Read the model definition and answer for the solid it produces. Units are mm, in the model's axes. A direction names the side the tool comes from. Round coordinates to 2 decimals unless told otherwise and drop trailing zeros. Order: outer loops, then holes, each group sorted by start corner. A loop starts at its lowest first (then second) coordinate and runs counter-clockwise, first axis right, second up. Notation, with made-up numbers: (42.5, 1) -> (61.5, 1) arc R31 ccw to (61.5, 28) -> close; hole circle Ø7 at (10, -7). An arc over 180 degrees is marked (long way). Use a Markdown table: item, result. Add a question column.
1. Section B-B, the plane z = -30 is taken. Give the vertices of the cut face in (x, y), then the cut area to 3 significant figures.
2. Section C-C, the plane y = 9 is taken. Give the vertices of the cut face in (x, z), then the cut area to 3 significant figures.
3. Section A-A, the plane y = 33 is taken. Give the vertices of the cut face in (x, z), then the cut area to 3 significant figures.
4. Consider L1, parallel to X at y = 61.5, z = -33.5; L2, parallel to Z at x = 115, y = 70.5; L3, parallel to Z at x = 97, y = 15.5. Determine where each line is inside the solid, lowest interval first. Write a range as [from, to].
5. The mould has two halves that part along X. Classify faces 5 (the face through (73.73, 13.72, -3.94)), 6 (the face through (116, -9, -33)), 7 (the face through (92.58, 13.72, -3.94)), 8 (the face through (45.675, 13.782, -3.944)): +X half, -X half, draft (parallel to the pull), parting line (faces both ways), or undercut.
6. Given pin 1 (1.4 mm diameter, centred on x = 47, z = -4.5, fed in from +Y); pin 2 (1 mm diameter, centred on y = 43.5, z = -56.5, fed in from -X); pin 3 (4 mm diameter, centred on x = 115.5, z = -13.5, fed in from +Y); pin 4 (12 mm diameter, centred on x = 90.5, z = -15, fed in from -Y), each flat-ended and moving along its own axis, determine where each tip first touches the part or whether it passes through.
7. For faces 1 (the face through (116, 10.5, -16)), 2 (the face through (83.374, 13.782, -3.944)), 3 (the face through (117.71, 13.72, -3.94)), 4 (the face through (116, 76, -103.5)), determine the directions among +Z, -Z, +X, -X, +Y, -Y from which every point of the face is accessible in a straight line to the end or side of a thin tool.
```python
from build123d import *

# Parameters (mm, degrees)
BLANKSKE_W          = 120
BLANKSKE_H          = 16
BLANK_DEPTH         = 8
TOOTHCUTSIM_DEPTH   = 122.326007105
TEETHCUTS_COUNT     = 20
TEETHCUTS_PITCH     = 6.2831853
SKETCH1_W           = 8
SKETCH1_H           = 1
CUT_EXTRUDE1_DEPTH  = 122.326007105
BOSS_EXTRUDE2_DEPTH = 8
CUT_EXTRUDE2_DEPTH  = 183.738200713


with BuildPart() as part:
    # BlankSke → Blank (new body)
    with BuildSketch(Plane.XY):
        with Locations((60, 8)):
            Rectangle(BLANKSKE_W, BLANKSKE_H)
    extrude(amount=-BLANK_DEPTH)

    # TooCutSkeSim → ToothCutSim (cut, through all)
    with BuildSketch(Plane.XY):
        Polygon((0.861870739, 11.5), (-0.861870739, 11.5), (-2.508981637, 16.0254), (2.508981637, 16.0254), align=None)
    toothcutsim = extrude(amount=-TOOTHCUTSIM_DEPTH, mode=Mode.SUBTRACT)

    # TeethCuts: ToothCutSim ×20
    with Locations(*[(i * TEETHCUTS_PITCH, 0, 0) for i in range(1, TEETHCUTS_COUNT)]):
        add(toothcutsim, mode=Mode.SUBTRACT)

    # Sketch1 → Cut-Extrude1 (cut, through all)
    with BuildSketch(Plane(origin=(120, 0, 0), x_dir=(0, 0, -1), z_dir=(1, 0, 0))):
        with Locations((4, 0.5)):
            Rectangle(SKETCH1_W, SKETCH1_H)
    extrude(amount=-CUT_EXTRUDE1_DEPTH, mode=Mode.SUBTRACT)

    # Sketch2 → Boss-Extrude2 (add)
    with BuildSketch(Plane(origin=(120, 0, 0), x_dir=(0, 0, -1), z_dir=(1, 0, 0))):
        Polygon((8, 1), (23.5, 1), (23.5, -9), (43.5, -9), (103.5, 61), (103.5, 91), (23.5, 91), (23.5, 10.5), (8, 10.5), align=None)
    extrude(amount=-BOSS_EXTRUDE2_DEPTH)

    # Sketch3 → Cut-Extrude2 (cut, through all)
    with BuildSketch(Plane.XY):
        with BuildLine():
            Line((0, 1), (0, 11.5))
            ThreePointArc((0, 11.5), (0.43093537, 11.93093537), (0.861870739, 11.5))
            Line((0.861870739, 11.5), (2.499736794, 16))
            Line((2.499736794, 16), (3.783448506, 16))
            Line((3.783448506, 16), (5.421314561, 11.5))
            Line((5.421314561, 11.5), (7.145056039, 11.5))
            Line((7.145056039, 11.5), (8.782922094, 16))
            Line((8.782922094, 16), (10.066633806, 16))
            Line((10.066633806, 16), (11.704499861, 11.5))
            Line((11.704499861, 11.5), (13.428241339, 11.5))
            Line((13.428241339, 11.5), (15.066107394, 16))
            Line((15.066107394, 16), (15.70796325, 16))
            Line((15.70796325, 16), (16.349819106, 16))
            Line((16.349819106, 16), (17.987685161, 11.5))
            Line((17.987685161, 11.5), (19.711426639, 11.5))
            Line((19.711426639, 11.5), (21.349292694, 16))
            Line((21.349292694, 16), (22.633004406, 16))
            Line((22.633004406, 16), (24.270870461, 11.5))
            Line((24.270870461, 11.5), (25.994611939, 11.5))
            Line((25.994611939, 11.5), (27.632477994, 16))
            Line((27.632477994, 16), (28.916189706, 16))
            Line((28.916189706, 16), (30.554055761, 11.5))
            Line((30.554055761, 11.5), (32.277797239, 11.5))
            Line((32.277797239, 11.5), (33.915663294, 16))
            Line((33.915663294, 16), (35.199375006, 16))
            Line((35.199375006, 16), (36.837241061, 11.5))
            Line((36.837241061, 11.5), (37.6991118, 11.5))
            Line((37.6991118, 11.5), (38.560982539, 11.5))
            Line((38.560982539, 11.5), (40.198848594, 16))
            Line((40.198848594, 16), (41.482560306, 16))
            Line((41.482560306, 16), (43.120426361, 11.5))
            Line((43.120426361, 11.5), (43.9822971, 11.5))
            Line((43.9822971, 11.5), (43.9822971, 1))
            Line((43.9822971, 1), (37.6991118, 1))
            Line((37.6991118, 1), (17.987685161, 1))
            Line((17.987685161, 1), (15.70796325, 1))
            Line((15.70796325, 1), (6.161314561, 1))
            Line((6.161314561, 1), (0, 1))
        make_face()
    extrude(amount=-CUT_EXTRUDE2_DEPTH, mode=Mode.SUBTRACT)


solid = part.part
```
Verdict:
| question | item | result |
|---|---|---|
| 1 | outline | (112, -9) -> (120, -9) -> (120, 91) -> (112, 91) -> close |
| 1 | area | 800 mm2 |
| 2 | outline | (43.98, -8) -> (112, -8) -> (112, -58.93) -> (120, -58.93) -> (120, 0) -> (43.98, 0) -> close |
| 2 | area | 1,020 mm2 |
| 3 | outline | (112, -79.5) -> (120, -79.5) -> (120, -23.5) -> (112, -23.5) -> close |
| 3 | area | 448 mm2 |
| 4 | L1 | x = [112, 120] |
| 4 | L2 | z = [-103.5, -23.5] |
| 4 | L3 | z = [-8, 0] |
| 5 | face 5 | undercut |
| 5 | face 6 | draft |
| 5 | face 7 | undercut |
| 5 | face 8 | -X half |
| 6 | pin 1 | stops at y = 16 |
| 6 | pin 2 | stops at x = 112 |
| 6 | pin 3 | stops at y = 10.5 |
| 6 | pin 4 | passes through |
| 7 | face 1 | +X, -X, +Y |
| 7 | face 2 | +Z, -Z, +Y |
| 7 | face 3 | +Z, +X, +Y |
| 7 | face 4 | -Z, +X, -X, +Y, -Y |
